The drawing under review shows one solid part. Ordinate dimensions are in mm from its lowest x, y, z. Coordinates: 2 decimals unless noted, no trailing zeros. Order: outer loops, then holes, each group sorted by start corner. A loop starts at its lowest first (then second) coordinate and runs counter-clockwise, first axis right, second up.
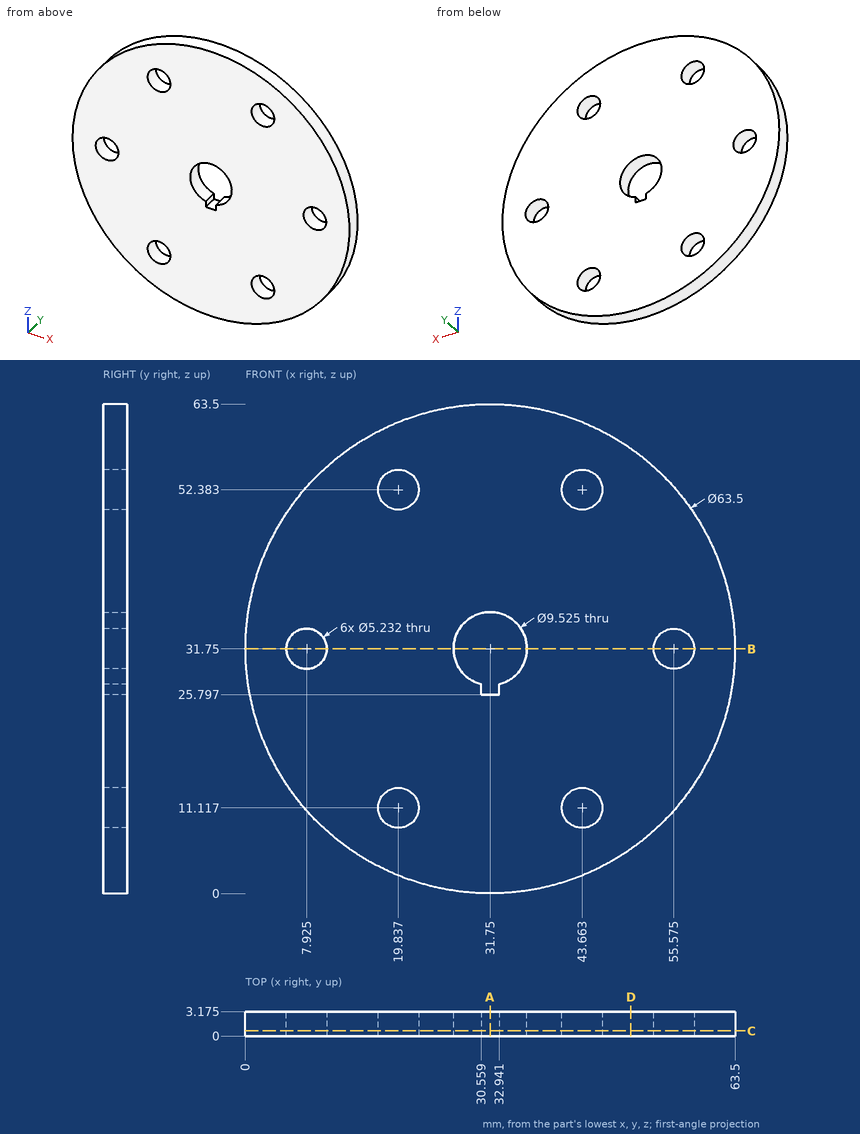
(1) We need section B-B, the plane z = 31.75. Write out the cut boundary in (x, y) (1 decimal), and give its area (3 significant figures).
A:
outline: (0, 0) - (5.3, 0) - (5.3, 3.2) - (0, 3.2) - close; (10.5, 0) - (27, 0) - (27, 3.2) - (10.5, 3.2) - close; (36.5, 0) - (53, 0) - (53, 3.2) - (36.5, 3.2) - close; (58.2, 0) - (63.5, 0) - (63.5, 3.2) - (58.2, 3.2) - close
area: 138 mm2
(2) We need section D-D, the plane x = 50. Write out the cut boundary in (y, z) (1 decimal), and give its area (3 significant figures).
A:
outline: (0, 5.8) - (3.2, 5.8) - (3.2, 57.7) - (0, 57.7) - close
area: 165 mm2
(3) Wall thickness on probe 1 along X at (y, z) = (3.05, 31.5) (1 decimal); probe 2 along X at (y, z) = (1.1, 30.5) (1 decimal); probe 3 along Z at (x, y) = (42, 1.45) (1 decimal): over which ranges is each line inside the solid? List them lowest first.
A:
probe 1: x = 0 to 5.3, 10.5 to 27, 36.5 to 53, 58.2 to 63.5
probe 2: x = 0 to 5.6, 10.2 to 27.2, 36.3 to 53.3, 57.9 to 63.5
probe 3: z = 1.7 to 9.1, 13.1 to 50.4, 54.4 to 61.8
(4) We need section A-A, the plane x = 31.75. Write out the cut boundary in (y, z) (1 decimal).
A:
outline: (0, 0) - (3.2, 0) - (3.2, 25.8) - (0, 25.8) - close; (0, 36.5) - (3.2, 36.5) - (3.2, 63.5) - (0, 63.5) - close
(5) For pin 1 Ø1 at (x, y) = (55.5, 2) entering from -Z; pin 2 Ø1.5 at (x, y) = (44, 2.5) entering from +Z (1 decimal); pin 3 Ø1.5 at (y, z) = (1.5, 26.5) entering from +X, all flat-tipped, find the tip position at first contact; note any pin that passes through.
A:
pin 1: stops at z = 10.13
pin 2: stops at z = 61.3
pin 3: stops at x = 63.18
(6) We need section C-C, the plane y = 0.65. Count the separate pieces of the cut face and the enclosed holes in it, and give its area (3 significant figures).
A:
separate pieces: 1
enclosed holes: 7
area: 2,960 mm2
